```python
from build123d import *

# Parameters (mm, degrees)
SKETCH1_W           = 12.5
SKETCH1_H           = 20
SKETCH2_R           = 10
BOSS_EXTRUDE1_DEPTH = 324
SKETCH3_R           = 9.75
BOSS_EXTRUDE2_DEPTH = 12.5
CUT_EXTRUDE1_START  = -8
CUT_EXTRUDE1_DEPTH  = 8
CUT_EXTRUDE2_START  = -8
CUT_EXTRUDE2_DEPTH  = 8
CUT_EXTRUDE3_START  = -8
CUT_EXTRUDE3_DEPTH  = 8
CUT_EXTRUDE4_START  = -8
CUT_EXTRUDE4_DEPTH  = 8
SKETCH8_R           = 7
BOSS_EXTRUDE3_DEPTH = 23.5
CHAMFER1_SIZE       = 0.92


with BuildPart() as part:
    # Sketch1 → Revolve1 (revolve)
    with BuildSketch(Plane.XZ, mode=Mode.PRIVATE) as revolve1_sk:
        with Locations((6.25, -332)):
            Rectangle(SKETCH1_W, SKETCH1_H)
    revolve(revolve1_sk.sketch.rotate(Axis((0, 0, -322), (0, 0, -1)), 180), axis=Axis((0, 0, -322), (0, 0, -1)))

    # Sketch2 → Boss-Extrude1 (add)
    with BuildSketch(Plane.XY.offset(-322)):
        Circle(SKETCH2_R)
    extrude(amount=BOSS_EXTRUDE1_DEPTH)

    # Sketch3 → Boss-Extrude2 (add)
    with BuildSketch(Plane.XY.offset(2)):
        Circle(SKETCH3_R)
    extrude(amount=BOSS_EXTRUDE2_DEPTH)

    # Sketch4 → Cut-Extrude1 (cut)
    with BuildSketch(Plane.XY.offset(14.5).offset(CUT_EXTRUDE1_START)):
        with BuildLine():
            Line((-8.5, -4.776243294), (-8.5, 4.776243294))
            ThreePointArc((-8.5, 4.776243294), (-9.75, 0), (-8.5, -4.776243294))
        make_face()
    extrude(amount=CUT_EXTRUDE1_DEPTH, mode=Mode.SUBTRACT)

    # Sketch5 → Cut-Extrude2 (cut)
    with BuildSketch(Plane.XY.offset(14.5).offset(CUT_EXTRUDE2_START)):
        with BuildLine():
            Line((4.776243294, -8.5), (-4.776243294, -8.5))
            ThreePointArc((-4.776243294, -8.5), (0, -9.75), (4.776243294, -8.5))
        make_face()
    extrude(amount=CUT_EXTRUDE2_DEPTH, mode=Mode.SUBTRACT)

    # Sketch6 → Cut-Extrude3 (cut)
    with BuildSketch(Plane.XY.offset(14.5).offset(CUT_EXTRUDE3_START)):
        with BuildLine():
            Line((8.5, 4.776243294), (8.5, -4.776243294))
            ThreePointArc((8.5, -4.776243294), (9.75, 0), (8.5, 4.776243294))
        make_face()
    extrude(amount=CUT_EXTRUDE3_DEPTH, mode=Mode.SUBTRACT)

    # Sketch7 → Cut-Extrude4 (cut)
    with BuildSketch(Plane.XY.offset(14.5).offset(CUT_EXTRUDE4_START)):
        with BuildLine():
            Line((-4.776243294, 8.5), (4.776243294, 8.5))
            ThreePointArc((4.776243294, 8.5), (0, 9.75), (-4.776243294, 8.5))
        make_face()
    extrude(amount=CUT_EXTRUDE4_DEPTH, mode=Mode.SUBTRACT)

    # Sketch8 → Boss-Extrude3 (add)
    with BuildSketch(Plane.XY.offset(14.5)):
        Circle(SKETCH8_R)
    extrude(amount=BOSS_EXTRUDE3_DEPTH)

    # Chamfer1
    chamfer1_edges = [part.edges().sort_by_distance(p)[0] for p in [
        (-7, 0, 38),
    ]]
    chamfer(chamfer1_edges, length=CHAMFER1_SIZE)


solid = part.part
```
The model under review builds one solid part; all positions refer to its coordinate system, in mm. A direction names the side the tool comes from. Round coordinates to 2 decimals unless told otherwise and drop trailing zeros. Loops run counter-clockwise (first coordinate to the right, second up) from the corner with the lowest first, then second, coordinate; pieces in that order, holes last.
1) Tool access review of faces 1 (the face through (8.5, 0, 10)), 2 (the face through (0, -8.5, 10)), 3 (the face through (6.466, -2.681, 25.632)), 4 (the face through (0, 8.5, 10)): name each direction out of +Z, -Z, +X, -X, +Y, -Y from which nothing blocks a thin tool from reaching the whole face with its end or side.
Values follow:
face 1: +Z, +X, +Y, -Y
face 2: +Z, +X, -X, -Y
face 3: +Z
face 4: +Z, +X, -X, +Y
2) Wall thickness on line 1 along Z through (x, y) = (-2, 7); line 2 along Z through (x, y) = (-5, 8.75); line 3 along X through (y, z) = (2.5, -18): over which ranges is each line inside the solid? List them lowest first.
Values follow:
line 1: z = -342 to 14.5
line 2: z = -342 to -322
line 3: x = -9.68 to 9.68
3) Clearance check with flat-ended pins moving along their axes: P1, Ø5, axis at x = 6, y = 3.5, coming from the +Z side; P2, Ø3, axis at x = 6, z = -53, coming from the +Y side; P3, Ø3, axis at x = -6.5, z = -102, coming from the -Y side; P4, Ø2.5, axis at y = 1, z = 10.5, coming from the +X side. State where each tip first meets the part, or that it passes through.
Values follow:
P1: stops at z = 38
P2: stops at y = 8.93
P3: stops at y = -8.66
P4: stops at x = 8.5
4) Consider section C-C on z = -277.5. State the section outline as (x, y) points.
Values follow:
outline: circle Ø20 at (0, 0)
5) Consider section A-A on x = 0. State the section outline as (y, z) points.
Values follow:
outline: (-12.5, -342) - (12.5, -342) - (12.5, -322) - (10, -322) - (10, 2) - (9.75, 2) - (9.75, 6.5) - (8.5, 6.5) - (8.5, 14.5) - (7, 14.5) - (7, 37.08) - (6.08, 38) - (-6.08, 38) - (-7, 37.08) - (-7, 14.5) - (-8.5, 14.5) - (-8.5, 6.5) - (-9.75, 6.5) - (-9.75, 2) - (-10, 2) - (-10, -322) - (-12.5, -322) - close
